The drawing under review shows one solid part. Ordinate dimensions are in mm from its lowest x, y, z. A direction names the side the tool comes from. Round coordinates to 2 decimals unless told otherwise and drop trailing zeros. Order: outer loops, then holes, each group sorted by start corner. A loop starts at its lowest first (then second) coordinate and runs counter-clockwise, first axis right, second up. Notation, with made-up numbers: (56.5, 40.5) - (75.5, 40.5) arc R14 ccw to (75.5, 50.5) - close; hole circle Ø11 at (-24.75, 25.5). An arc over 180 degrees is marked (long way). One line per question, with ' | ' between items.
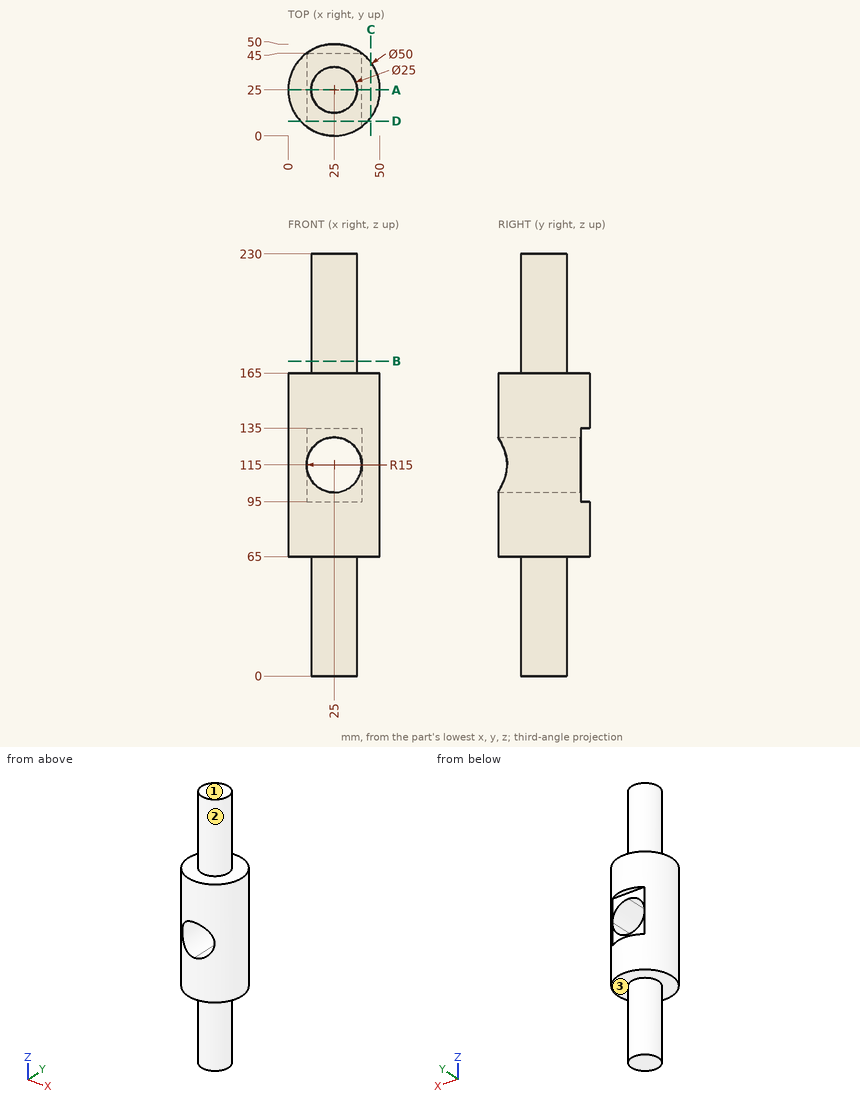
(1) We need section C-C on x = 45. State the section outline as (y, z) points, plus the area to 3 significant figures.
Output values:
outline: (10, 65) - (40, 65) - (40, 165) - (10, 165) - close | area: 3,000 mm^2
(2) For probe 1 along Y at (x, z) = (5, 136); probe 2 along Z at (x, y) = (46, 31.5); probe 3 along Z at (x, y) = (21, 31), list the stretches that pass through material, from the lowest coordinate up. Write a range as [from, to].
Output values:
probe 1: [10, 40] | probe 2: [65, 165] | probe 3: [0, 100.54], [129.46, 230]
(3) Insertion check: pin 1 (12 mm diameter, centred on y = 16.5, z = 117.5, fed in from -X); pin 2 (5 mm diameter, centred on x = 32.5, z = 101, fed in from +Y); pin 3 (12 mm diameter, centred on y = 22.5, z = 180, fed in from +X); pin 4 (16 mm diameter, centred on x = 25, z = 109.5, fed in from +Y). Each pin has a flat end and moves straight along its axis. Give the tip position at first contact, or say it passes through.
Output values:
pin 1: x = 0.13 | pin 2: y = 45 | pin 3: x = 37.5 | pin 4: through
(4) For the marked faces 1, 2 and 3, list the 3-axis set-ups (+Z, -Z, +X, -X, +Y, -Y) from which the entire face can be reached by the end or side of a thin tool; tool diameter is ignored.
Output values:
face 1: +Z, +X, -X, +Y, -Y | face 2: +Z | face 3: -Z
(5) We need section A-A on y = 25. State the section outline as (x, z) points.
Output values:
outline: (0, 65) - (12.5, 65) - (12.5, 0) - (37.5, 0) - (37.5, 65) - (50, 65) - (50, 165) - (37.5, 165) - (37.5, 230) - (12.5, 230) - (12.5, 165) - (0, 165) - close; hole circle Ø30 at (25, 115)
(6) We need section B-B on z = 171.5. State the section outline as (x, y) points, plus the area to 3 significant figures.
Output values:
outline: circle Ø25 at (25, 25) | area: 491 mm^2
(7) We need section D-D on y = 8. State the section outline as (x, z) points.
Output values:
outline: (6.67, 65) - (43.33, 65) - (43.33, 165) - (6.67, 165) - close; hole circle Ø30 at (25, 115)
